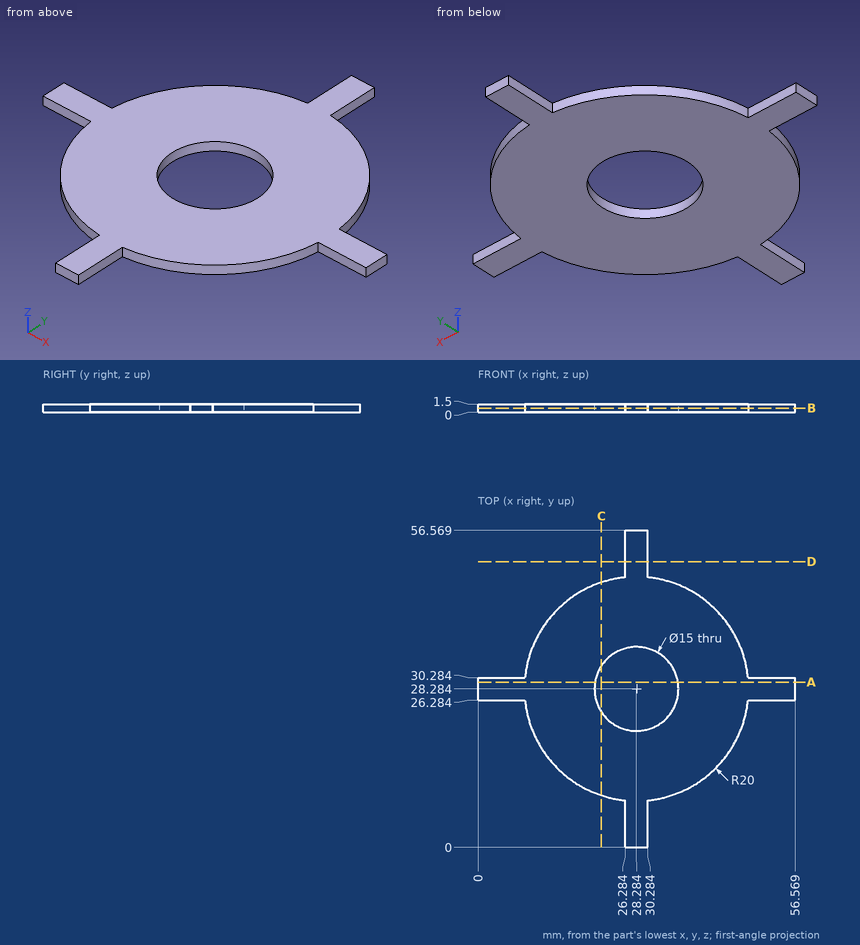
The figure shows three views and two pictorial views of one solid part (mm, origin at its lowest corner). Answer the questions. Coordinates: 2 decimals unless noted, no trailing zeros. Loops run counter-clockwise (first coordinate to the right, second up) from the corner with the lowest first, then second, coordinate; pieces in that order, holes last. Notation, with made-up numbers: (67, 17) -> (103, 17) arc R20 ccw to (103, 56) -> close; hole circle Ø8 at (-15, -14). An arc over 180 degrees is marked (long way). Return JSON: item names as keys, results as strings. Group by question number.
(1) A cutting plane is placed at A-A on y = 29.5. Write down the section's boundary in (x, z) (1 decimal).
(2) A cutting plane is placed at B-B on z = 0.75. Write down the section's boundary in (x, y) (1 decimal), and give its area (3 significant figures).
(3) A cutting plane is placed at C-C on x = 22. Write down the section's boundary in (y, z).
(4) Find the intervals of material crossed by probe 1 along Y at (x, z) = (31.5, 0.9) (1 decimal); probe 2 along Y at (x, z) = (25, 1.3) (1 decimal); probe 3 along X at (y, z) = (53.5, 0.1) (1 decimal), in increasing order. Write a range as from..to.
(5) A cutting plane is placed at D-D on y = 51. Write down the section's boundary in (x, z) (1 decimal).
(6) Given pin 1 Ø10 at (x, y) = (12.5, 8) entering from -Z; pin 2 Ø0.8 at (x, z) = (53.5, 0.5) entering from -Y, each flat-ended and moving along its own axis, determine where each tip first touches the part or whether it passes through.
The answers:
{
 "1": {"outline": "(0, 0) -> (20.9, 0) -> (20.9, 1.5) -> (0, 1.5) -> close; (35.7, 0) -> (56.6, 0) -> (56.6, 1.5) -> (35.7, 1.5) -> close"},
 "2": {"outline": "(0, 26.3) -> (8.4, 26.3) arc R20 ccw to (26.3, 8.4) -> (26.3, 0) -> (30.3, 0) -> (30.3, 8.4) arc R20 ccw to (48.2, 26.3) -> (56.6, 26.3) -> (56.6, 30.3) -> (48.2, 30.3) arc R20 ccw to (30.3, 48.2) -> (30.3, 56.6) -> (26.3, 56.6) -> (26.3, 48.2) arc R20 ccw to (8.4, 30.3) -> (0, 30.3) -> close; hole circle Ø15 at (28.3, 28.3)", "area": "1,210 mm^2"},
 "3": {"outline": "(9.3, 0) -> (24.19, 0) -> (24.19, 1.5) -> (9.3, 1.5) -> close; (32.38, 0) -> (47.27, 0) -> (47.27, 1.5) -> (32.38, 1.5) -> close"},
 "4": {"probe 1": "y = 8.5..21.5, 35.1..48", "probe 2": "y = 8.6..21.5, 35..48", "probe 3": "x = 26.3..30.3"},
 "5": {"outline": "(26.3, 0) -> (30.3, 0) -> (30.3, 1.5) -> (26.3, 1.5) -> close"},
 "6": {"pin 1": "passes through", "pin 2": "stops at y = 26.28"}
}
